Answer from the drawing. Dimensions are ordinates in mm from the lowest x, y and z of the part. A direction names the side the tool comes from. Coordinates: 2 decimals unless noted, no trailing zeros. Loops run counter-clockwise (first coordinate to the right, second up) from the corner with the lowest first, then second, coordinate; pieces in that order, holes last. Notation, with made-up numbers: (37, -11.5) -> (55, -11.5) arc R20 cw to (55, 20.5) -> close; hole circle Ø11 at (75, 25). An arc over 180 degrees is marked (long way). Answer as CSV lines item,"result".
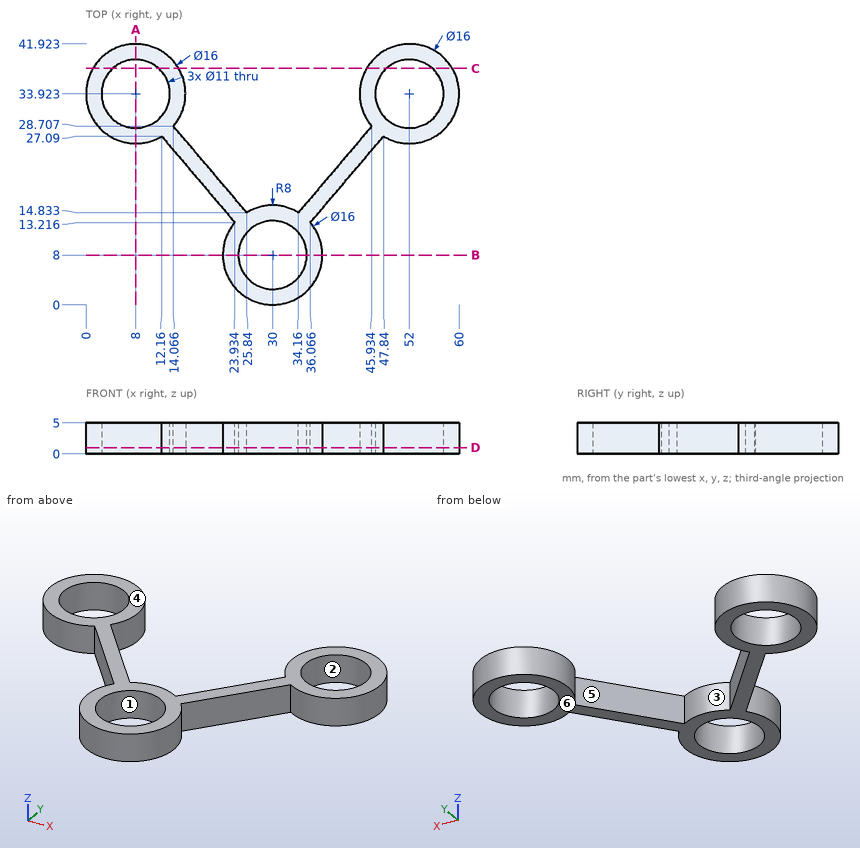
(1) A cutting plane is placed at C-C, the plane y = 38. Write down the section's boundary in (x, z).
Computed values:
outline,"(1.12, 0) -> (4.31, 0) -> (4.31, 5) -> (1.12, 5) -> close; (11.69, 0) -> (14.88, 0) -> (14.88, 5) -> (11.69, 5) -> close; (45.12, 0) -> (48.31, 0) -> (48.31, 5) -> (45.12, 5) -> close; (55.69, 0) -> (58.88, 0) -> (58.88, 5) -> (55.69, 5) -> close"
(2) Which of the six approach directions +Z, -Z, +X, -X, +Y, -Y give full straight-line access (tool end or side, diameter ignored) to the marked faces 5 and 6?
Computed values:
face 5,"+Z, -Z"
face 6,"-Z, +X, -X, +Y, -Y"
(3) Consider line 1 along Y through (x, z) = (30, 2.6); line 2 along Y through (x, z) = (52, 3.95); line 3 along X through (y, z) = (38, 1.8) (1 decimal). Determine where each line is inside the solid, lowest interval first.
Computed values:
line 1,"0 to 2.5, 13.5 to 16"
line 2,"25.92 to 28.42, 39.42 to 41.92"
line 3,"1.1 to 4.3, 11.7 to 14.9, 45.1 to 48.3, 55.7 to 58.9"
(4) For a pull along Y with two mould halves and no side action, classify the marked faces 1, 2, 3 and 4 as pulls with the +Y half, pulls with the -Y half, needs draft (parallel to the pull), parting line crosses it, or undercut.
Computed values:
face 1,"undercut"
face 2,"undercut"
face 3,"pulls with the +Y half"
face 4,"needs draft"
(5) Flat-ended cylindrical pins translate along their axes: pin 1 Ø1.5 at (x, z) = (6.5, 3.5) entering from +Y; pin 2 Ø10 at (x, y) = (8, 33.92) entering from +Z; pin 3 Ø1 at (x, z) = (9.5, 4) entering from -Y. Find the tip coordinate at first contact, or state that the pin passes through.
Computed values:
pin 1,"y = 41.89"
pin 2,"through"
pin 3,"y = 25.99"
(6) A cutting plane is placed at D-D, the plane z = 1. Write down the section's boundary in (x, y) (1 decimal).
Computed values:
outline,"(12.2, 27.1) -> (23.9, 13.2) arc R8 ccw (long way) to (36.1, 13.2) -> (47.8, 27.1) arc R8 ccw (long way) to (45.9, 28.7) -> (34.2, 14.8) arc R8 ccw to (25.8, 14.8) -> (14.1, 28.7) arc R8 ccw (long way) to start; hole circle Ø11 at (8, 33.9); hole circle Ø11 at (30, 8); hole circle Ø11 at (52, 33.9)"
(7) A cutting plane is placed at B-B, the plane y = 8. Write down the section's boundary in (x, z).
Computed values:
outline,"(22, 0) -> (24.5, 0) -> (24.5, 5) -> (22, 5) -> close; (35.5, 0) -> (38, 0) -> (38, 5) -> (35.5, 5) -> close"
(8) A cutting plane is placed at A-A, the plane x = 8. Write down the section's boundary in (y, z).
Computed values:
outline,"(25.92, 0) -> (28.42, 0) -> (28.42, 5) -> (25.92, 5) -> close; (39.42, 0) -> (41.92, 0) -> (41.92, 5) -> (39.42, 5) -> close"
